Geometry check sheet. Reference: drawing and pictorial views, mm from the part's lowest x, y, z. A direction names the side the tool comes from. Give positions to 0.01 mm unless a question says otherwise; leave off trailing zeros. Loops run counter-clockwise (first coordinate to the right, second up) from the corner with the lowest first, then second, coordinate; pieces in that order, holes last. Notation, with made-up numbers: M 82.25,-1.75 L 103.25,-1.75 A26 ccw 103.25,20.25 Z; hole C 5.5,-10.75 d6. An arc over 180 degrees is marked long. Use CSV: the item, a comma, the result in double quotes.
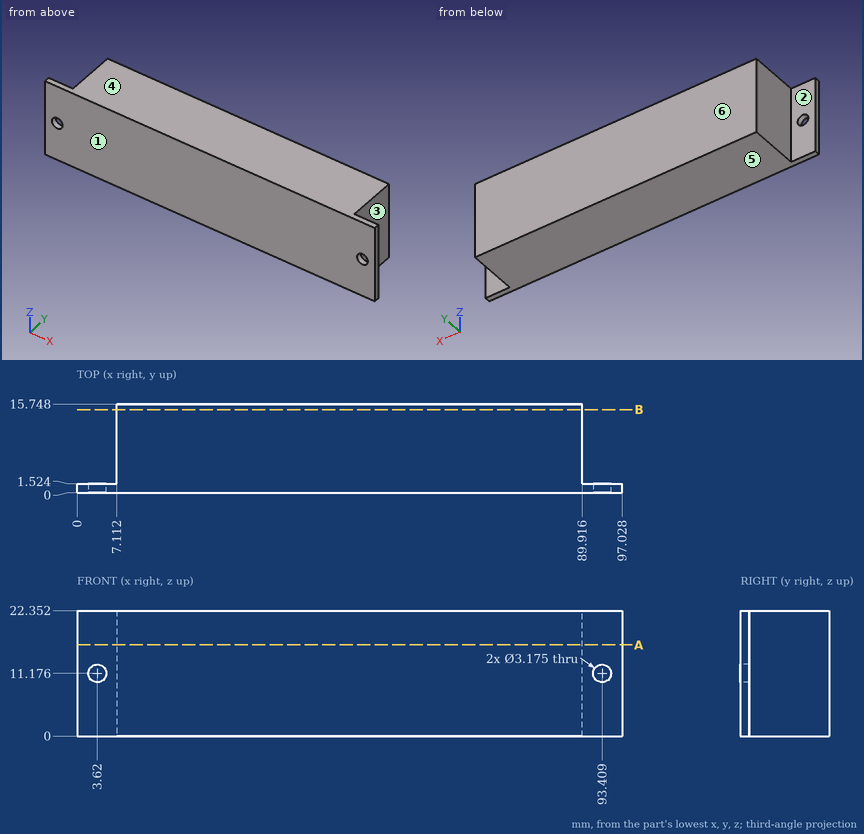
(1) Depth check by flat-ended pin: pin 1 Ø3.5 at (x, z) = (2, 15.5) entering from +Y. Enter the tip coordinate at first touch or a pass-through.
Calculated:
pin 1,"stops at y = 1.52"
(2) Section check B-B on y = 14.75. Record the cut outline in (x, z) (1 decimal).
Calculated:
outline,"M 7.1,0 L 89.9,0 L 89.9,22.4 L 7.1,22.4 Z"
(3) Scan lines: L1, parallel to X at y = 2.5, z = 11 (1 decimal); L2, parallel to Y at x = 6.5, z = 9.25 (1 decimal). Record each from-to range of solid material in increasing order. Write a range as from..to.
Calculated:
L1,"x = 7.1..89.9"
L2,"y = 0..1.5"
(4) Tool access check on the marked faces 1, 2 and 3. Record the directions out of +Z, -Z, +X, -X, +Y, -Y that give a thin tool (end or side, any length) a straight path to the whole face; none if there is none.
Calculated:
face 1,"+Z, -Z, +X, -X, -Y"
face 2,"+Z, -Z, -X, +Y"
face 3,"+Z, -Z, +X, +Y"
(5) Mould release check, pull along Z, two halves, no side actions. Record for the marked faces 4, 5 and 6: released by +Z, released by -Z, zero draft, split by the parting line, or undercut.
Calculated:
face 4,"released by +Z"
face 5,"released by -Z"
face 6,"zero draft"
(6) Section check A-A on z = 16.25. Record the cut outline in (x, y) (1 decimal), plus the area to 3 significant figures.
Calculated:
outline,"M 0,0 L 97,0 L 97,1.5 L 89.9,1.5 L 89.9,15.7 L 7.1,15.7 L 7.1,1.5 L 0,1.5 Z"
area,"1,330 mm²"
